Model file for the job. Use its own axes, mm. A direction names the side the tool comes from. Round coordinates to 2 decimals unless told otherwise and drop trailing zeros. Loops run counter-clockwise (first coordinate to the right, second up) from the corner with the lowest first, then second, coordinate; pieces in that order, holes last. Notation, with made-up numbers: (16.25, 43) -> (38.25, 43) arc R23 ccw to (38.25, 65) -> close; hole circle Ø7 at (84, 73). An arc over 180 degrees is marked (long way). Use a Markdown table: item, result.
from build123d import *

# Parameters (mm, degrees)
F1_DEPTH      = 5
F2_W          = 10
F2_H          = 10
F3_DEPTH      = 5.001
F3_DEPTH_BACK = 5.001


with BuildPart() as f1:
    # F0 (on Right) → F1 (new body, symmetric)
    with BuildSketch(Plane.YZ):
        with BuildLine():
            Line((8.7534596749, 22.0049817023), (7.8275281652, 22.3511091184))
            ThreePointArc((7.8275281652, 22.3511091184), (3.3739717902, 19.8784451352), (0.2100715875, 15.8862067822))
            ThreePointArc((0.2100715875, 15.8862067822), (-0.1018352129, 15.4564251276), (-0.5296881322, 15.1418778303))
            ThreePointArc((-0.5296881322, 15.1418778303), (-0.9784750701, 15.4257588038), (-1.3196516389, 15.8326945133))
            ThreePointArc((-1.3196516389, 15.8326945133), (-4.754786797, 19.5940876069), (-9.3702410866, 21.7495024766))
            Line((-9.3702410866, 21.7495024766), (-10.2697225791, 21.3395190702))
            ThreePointArc((-10.2697225791, 21.3395190702), (-11.6704250222, 16.4419416869), (-11.084701499, 11.3817875871))
            ThreePointArc((-11.084701499, 11.3817875871), (-11.0013513902, 10.857334651), (-11.0814705639, 10.3323784235))
            ThreePointArc((-11.0814705639, 10.3323784235), (-11.5995450124, 10.2157722978), (-12.1285402775, 10.2622710322))
            ThreePointArc((-12.1285402775, 10.2622710322), (-17.2172542053, 10.4929702308), (-22.0049817023, 8.7534596749))
            Line((-22.0049817023, 8.7534596749), (-22.3511091184, 7.8275281652))
            ThreePointArc((-22.3511091184, 7.8275281652), (-19.8784451352, 3.3739717902), (-15.8862067822, 0.2100715875))
            ThreePointArc((-15.8862067822, 0.2100715875), (-15.4564251276, -0.1018352129), (-15.1418778303, -0.5296881322))
            ThreePointArc((-15.1418778303, -0.5296881322), (-15.4257588038, -0.9784750701), (-15.8326945133, -1.3196516389))
            ThreePointArc((-15.8326945133, -1.3196516389), (-19.5940876069, -4.754786797), (-21.7495024766, -9.3702410866))
            Line((-21.7495024766, -9.3702410866), (-21.3395190702, -10.2697225791))
            ThreePointArc((-21.3395190702, -10.2697225791), (-16.4419416869, -11.6704250222), (-11.3817875871, -11.084701499))
            ThreePointArc((-11.3817875871, -11.084701499), (-10.857334651, -11.0013513902), (-10.3323784235, -11.0814705639))
            ThreePointArc((-10.3323784235, -11.0814705639), (-10.2157722978, -11.5995450124), (-10.2622710322, -12.1285402775))
            ThreePointArc((-10.2622710322, -12.1285402775), (-10.4929702308, -17.2172542053), (-8.7534596749, -22.0049817023))
            Line((-8.7534596749, -22.0049817023), (-7.8275281652, -22.3511091184))
            ThreePointArc((-7.8275281652, -22.3511091184), (-3.3739717902, -19.8784451352), (-0.2100715875, -15.8862067822))
            ThreePointArc((-0.2100715875, -15.8862067822), (0.1018352129, -15.4564251276), (0.5296881322, -15.1418778303))
            ThreePointArc((0.5296881322, -15.1418778303), (0.9784750701, -15.4257588038), (1.3196516389, -15.8326945133))
            ThreePointArc((1.3196516389, -15.8326945133), (4.754786797, -19.5940876069), (9.3702410866, -21.7495024766))
            Line((9.3702410866, -21.7495024766), (10.2697225791, -21.3395190702))
            ThreePointArc((10.2697225791, -21.3395190702), (11.6704250222, -16.4419416869), (11.084701499, -11.3817875871))
            ThreePointArc((11.084701499, -11.3817875871), (11.0013513902, -10.857334651), (11.0814705639, -10.3323784235))
            ThreePointArc((11.0814705639, -10.3323784235), (11.5995450124, -10.2157722978), (12.1285402775, -10.2622710322))
            ThreePointArc((12.1285402775, -10.2622710322), (17.2172542053, -10.4929702308), (22.0049817023, -8.7534596749))
            Line((22.0049817023, -8.7534596749), (22.3511091184, -7.8275281652))
            ThreePointArc((22.3511091184, -7.8275281652), (19.8784451352, -3.3739717902), (15.8862067822, -0.2100715875))
            ThreePointArc((15.8862067822, -0.2100715875), (15.4564251276, 0.1018352129), (15.1418778303, 0.5296881322))
            ThreePointArc((15.1418778303, 0.5296881322), (15.4257588038, 0.9784750701), (15.8326945133, 1.3196516389))
            ThreePointArc((15.8326945133, 1.3196516389), (19.5940876069, 4.754786797), (21.7495024766, 9.3702410866))
            Line((21.7495024766, 9.3702410866), (21.3395190702, 10.2697225791))
            ThreePointArc((21.3395190702, 10.2697225791), (16.4419416869, 11.6704250222), (11.3817875871, 11.084701499))
            ThreePointArc((11.3817875871, 11.084701499), (10.857334651, 11.0013513902), (10.3323784235, 11.0814705639))
            ThreePointArc((10.3323784235, 11.0814705639), (10.2157722978, 11.5995450124), (10.2622710322, 12.1285402775))
            ThreePointArc((10.2622710322, 12.1285402775), (10.4929702308, 17.2172542053), (8.7534596749, 22.0049817023))
        make_face()
    extrude(amount=F1_DEPTH, both=True)

    # F2 (on Right) → F3 (cut, two sides)
    with BuildSketch(Plane.YZ) as f3_sk:
        Rectangle(F2_W, F2_H)
    extrude(amount=-F3_DEPTH, mode=Mode.SUBTRACT)
    extrude(f3_sk.sketch, amount=F3_DEPTH_BACK, mode=Mode.SUBTRACT)


solid = f1.part
Q1. Band-saw the part on A-A, the plane z = -2. Give the cut face in (x, y) (3 decimals).
Results list:
| item | result |
|---|---|
| outline | (-5, -16.848) -> (5, -16.848) -> (5, -5) -> (-5, -5) -> close; (-5, 5) -> (5, 5) -> (5, 18.525) -> (-5, 18.525) -> close |
Q2. Band-saw the part on B-B, the plane y = 3. Give the cut face in (x, z).
Results list:
| item | result |
|---|---|
| outline | (-5, -18.04) -> (5, -18.04) -> (5, -5) -> (-5, -5) -> close; (-5, 5) -> (5, 5) -> (5, 19.55) -> (-5, 19.55) -> close |
Q3. Pull direction Z, two halves, no side cores. Call faces 1 (the face through (0.07, -10.504, -17.146)), 2 (the face through (0.07, -17.146, 10.504)), 3 (the face through (0.07, 4.697, -19.551)), 4 (the face through (0.07, 11, -10.86)): released by +Z, released by -Z, zero draft, split by the parting line, or undercut.
Results list:
| item | result |
|---|---|
| face 1 | undercut |
| face 2 | released by +Z |
| face 3 | released by -Z |
| face 4 | undercut |
Q4. Flat gauge pins, fed straight in: pin 1 (6 mm diameter, centred on x = -2.5, y = 1, fed in from +Z); pin 2 (5 mm diameter, centred on x = -2, y = 0.5, fed in from -Z) (3 decimals); pin 3 (1 mm diameter, centred on x = -3, y = -0.5, fed in from -Z). Where does each tip first touch, or does it go through?
Results list:
| item | result |
|---|---|
| pin 1 | stops at z = 20.38 |
| pin 2 | stops at z = -18.525 |
| pin 3 | stops at z = -17.23 |
Q5. Drill centre lines: L1, parallel to Z at x = -1.5, y = -20; L2, parallel to Z at x = -1.75, y = 4; L3, parallel to Y at x = -2.25, z = 4.5. Where is each one in solid material? Low to high. Write a range as from..to.
Results list:
| item | result |
|---|---|
| L1 | z = -10.87..-5.34, 3.52..9.75 |
| L2 | z = -19..-5, 5..20.38 |
| L3 | y = -20.73..-5, 5..19.4 |
Q6. Band-saw the part on D-D, the plane z = -6.5. Give the cut face in (x, y).
Results list:
| item | result |
|---|---|
| outline | (-5, -20.68) -> (5, -20.68) -> (5, 21.84) -> (-5, 21.84) -> close |
Q7. Band-saw the part on C-C, the plane z = -13. Give the cut face in (x, y), plus the area to 3 significant figures.
Results list:
| item | result |
|---|---|
| outline | (-5, -10.45) -> (5, -10.45) -> (5, 11.49) -> (-5, 11.49) -> close |
| area | 219 mm² |
Q8. Tool access for faces 5 (the face through (0.07, -4.697, 19.551)), 6 (the face through (0.07, 10.216, 11.592)), 7 (the face through (0.1, -19.9, 3.4)), 8 (the face through (0.07, 17.146, -10.504)), 9 (the face through (-5, -0.3, 5.3)): list every direction of +Z, -Z, +X, -X, +Y, -Y with a clear straight run to the whole face (end or side of a thin tool).
Results list:
| item | result |
|---|---|
| face 5 | +Z, +X, -X |
| face 6 | +X, -X |
| face 7 | +X, -X, -Y |
| face 8 | -Z, +X, -X |
| face 9 | +Z, -Z, -X, +Y, -Y |
